Geometry: final body of the model. Coordinates: model frame, mm. A direction names the side the tool comes from. Give positions to 0.01 mm unless a question says otherwise; leave off trailing zeros. Write each loop counter-clockwise with the first axis right and the second up, starting at its lowest first coordinate (ties: lowest second). Pieces come first, ordered by that corner, then holes. Notation, with made-up numbers: M -15.5,32 L -8.5,32 A26 ccw -8.5,59 Z; hole C 80.5,39 d10. An arc over 180 degrees is marked long. Use a Markdown table: item, result. Add a question column.
1) Section B-B on z = 2.75. Return the cut outline in (x, y), then the cut area to 3 significant figures.
2) Pin query (flat end, axial travel): pin 1 (0.6 mm diameter, centred on x = -30, z = 11.5, fed in from +Y) (3 decimals); pin 2 (12 mm diameter, centred on x = -4.5, z = 7, fed in from -Y); pin 3 (0.9 mm diameter, centred on x = -22.5, z = 18.5, fed in from +Y); pin 4 (2.5 mm diameter, centred on y = 6, z = 16.5, fed in from -X). Return the tip coordinate at first contact, or that it passes through.
3) Line query: line 1 (Z direction, x = -24.95, y = 6.5); line 2 (Z direction, x = -2.75, y = 4.5); line 3 (X direction, y = 6.5, z = 13). Output: solid intervals per line, ascending.
4) Section C-C on x = -2.75. Return the cut outline in (y, z), then the cut area to 3 significant figures.
5) Draft query along Z for faces 4 (the flat face through (-8.25, 5, -1)), 5 (the flat face through (-21, 5, 19.05)), 6 (the cylindrical face through (-2.425, 5.053, 14.514)). Return one class per face: +Z half, -Z half, draft (parallel to the pull), parting line (faces both ways), or undercut.
6) Section D-D on y = 1.5. Return the cut outline in (x, z), then the cut area to 3 significant figures.
7) Section A-A on x = -24.95. Return the cut outline in (y, z), then the cut area to 3 significant figures.
8) Set-up query: faces 1 (the flat face through (-31.7, 8.7, 11.4)), 2 (the flat face through (-16, 9.125, 18)), 3 (the flat face through (-35.6, 1.95, 11.4)). Return all of +Z, -Z, +X, -X, +Y, -Y with unobstructed straight access to the full face (end or side cutting, diameter ignored); none if empty.
Autodesk Inventor part; units mm, degrees
ref_plane "YZ Plane" through (0, 0, 0) normal (1, 0, 0) x (0, 1, 0)
ref_plane "XZ Plane" through (0, 0, 0) normal (0, 1, 0) x (-1, 0, 0)
ref_plane "XY Plane" through (0, 0, 0) normal (0, 0, 1) x (1, 0, 0)
sketch "Sketch1" plane through (0, 0, 0) normal (0, 1, 0) x (-1, 0, 0)
  circle A0 centre (2.75, 13.05) radius 1.5
  circle A1 centre (24.95, 2.75) radius 1.5
  line L0 (2, 15.8) -> (25.7, 15.8)
  line L1 (27.7, 13.8) -> (27.7, 2)
  line L2 (25.7, 0) -> (2, 0)
  line L3 (0, 2) -> (0, 13.8)
  arc A2 (0, 2) -> (2, 0) centre (2, 2) ccw
  arc A3 (25.7, 0) -> (27.7, 2) centre (25.7, 2) ccw
  arc A4 (27.7, 13.8) -> (25.7, 15.8) centre (25.7, 13.8) ccw
  arc A5 (2, 15.8) -> (0, 13.8) centre (2, 13.8) ccw
  point P0 (0, 0)
  point P1 (0, 0)
  point P2 (0, 0)
  dimension "d0" = 10.3
  dimension "d1" = 22.2
  dimension "d2" = 2.75
  dimension "d3" = 2.75
  dimension "d4" = 2.75
  dimension "d5" = 2.75
  dimension "d6" = 3
  dimension "d7" = 2
extrude "Extrusion1" add sketch "Sketch1" along normal blind 10.25
sketch "Sketch2" plane through (-2, 0, 0) normal (0, 0, -1) x (-1, 0, 0)
  line L0 (0, 0) -> (23.7, 0)
  line L1 (0, 10.25) -> (23.7, 10.25)
  line L2 (0, 0) -> (0, 10.25)
  line L3 (3.5, 7.25) -> (6.25, 7.25)
  line L4 (6.25, 7.25) -> (6.25, 3)
  line L5 (6.25, 3) -> (3.5, 3)
  line L6 (3.5, 3) -> (3.5, 7.25)
  point P0 (-2, 0)
  dimension "d10" = 4.25
  dimension "d12" = 2.75
  dimension "d13" = 3
  dimension "d14" = 3
  dimension "d15" = 3.5
extrude "Extrusion2" add sketch "Sketch2" along normal blind 2.5
sketch "Sketch3" plane through (-27.7, 0, 2) normal (-1, 0, 0) x (0, 0, 1)
  line L0 (0, 0) -> (11.8, 0)
  line L1 (0, 10.25) -> (11.8, 10.25)
  line L2 (9, 9.125) -> (9.8, 9.125)
  line L3 (9.8, 9.125) -> (9.8, 1.125)
  line L4 (9.8, 1.125) -> (9, 1.125)
  line L5 (9, 1.125) -> (9, 9.125)
  line L6 (-2, 0) -> (-2, 10.25)
  dimension "d18" = 8
  dimension "d20" = 0.8
  dimension "d21" = 1.125
  dimension "d22" = 1.125
  dimension "d23" = 11
extrude "Extrusion3" add sketch "Sketch3" along normal blind 12
sketch "Sketch5" plane through (-25.7, 0, 15.8) normal (0, 0, 1) x (1, 0, 0)
  line L0 (0, 0) -> (23.7, 0)
  line L1 (23.7, 0) -> (23.7, 10.25)
  line L2 (0, 10.25) -> (23.7, 10.25)
  line L3 (9.5, 9.125) -> (10.3, 9.125)
  line L4 (10.3, 9.125) -> (10.3, 1.125)
  line L5 (10.3, 1.125) -> (9.5, 1.125)
  line L6 (9.5, 1.125) -> (9.5, 9.125)
  line L7 (0, 0) -> (0, 10.25)
  point P0 (25.7, 0)
  dimension "d29" = 8
  dimension "d31" = 0.8
  dimension "d33" = 1.125
  dimension "d34" = 1.125
  dimension "d49" = 9.5
  dimension "d50" = 13.4
extrude "Extrusion5" add sketch "Sketch5" along normal blind 3.25 contours L3 L4 L5 L6
sketch "Sketch6" plane through (-15.4, 1.125, 15.8) normal (1, 0, 0) x (0, 0, -1)
  line L0 (0, 0) -> (-3.25, 0)
  line L1 (-3.25, 8) -> (-2.45, 8)
  line L2 (-2.45, 8) -> (-2.45, 0)
  line L3 (-2.45, 0) -> (-3.25, 0)
  line L4 (-3.25, 0) -> (-3.25, 8)
  point P0 (15.8, -1.125)
  dimension "d37" = 0.8
extrude "Extrusion6" add sketch "Sketch6" against normal blind 11
fillet "Fillet1" radius 1 1 edges at (-15.4, 5.125, 19.05)
fillet "Fillet2" radius 0.25 1 edges at (-16.2, 5.125, 18.25)
sketch "Sketch9" plane through (-25.7, 0, 19.05) normal (0, 0, 1) x (1, 0, 0)
  line L0 (9.3, 9.125) -> (-0.7, 9.125)
  line L1 (-0.7, 1.125) -> (-0.7, 9.125)
  line L2 (9.3, 1.125) -> (-0.7, 1.125)
  line L3 (7.3, 9.125) -> (7.3, 8.3)
  line L4 (7.3, 8.3) -> (-0.7, 8.3)
  line L5 (7.3, 1.125) -> (7.3, 1.95)
  line L6 (7.3, 1.95) -> (-0.7, 1.95)
  line L7 (10.3, 1.125) -> (10.3, 9.125)
  point P0 (25.7, 0)
  dimension "d51" = 6.35
  dimension "d53" = 3
extrude "Extrusion9" cut sketch "Sketch9" against normal up to next
sketch "Sketch10" plane through (-27.7, 1.125, 11.8) normal (0, 0, 1) x (1, 0, 0)
  line L0 (0, 8) -> (-12, 8)
  line L1 (-12, 0) -> (-12, 8)
  line L2 (0, 0) -> (-12, 0)
  line L3 (-12, 7.175) -> (-4, 7.175)
  line L4 (-4, 7.175) -> (-4, 8)
  line L5 (-4, 0) -> (-4, 0.825)
  line L6 (-4, 0.825) -> (-12, 0.825)
  point P0 (27.7, -1.125)
  dimension "d56" = 6.35
  dimension "d57" = 8
extrude "Extrusion10" cut sketch "Sketch10" against normal up to next
equation "\"d3\" = d2"
equation "\"d4\" = d2"
equation "\"d5\" = d2"
equation "\"d13\" = d14"
equation "\"d21\" = d22"
equation "\"d33\" = d34"
properties part number "EndStop_LimitSwitch"
Found:
| question | item | result |
|---|---|---|
| 1 | outline | M -27.7,0 L -26.45,0 L -26.45,10.25 L -27.7,10.25 Z; M -23.45,0 L 0,0 L 0,10.25 L -23.45,10.25 Z |
| 1 | area | 253 mm² |
| 2 | pin 1 | y = 9.125 |
| 2 | pin 2 | y = 0 |
| 2 | pin 3 | y = 8.3 |
| 2 | pin 4 | x = -27.08 |
| 3 | line 1 | 0 to 1.25, 4.25 to 15.8, 18.25 to 19.05 |
| 3 | line 2 | 0 to 11.55, 14.55 to 15.8 |
| 3 | line 3 | -27.7 to -4.25, -1.25 to 0 |
| 4 | outline | M 0,0 L 10.25,0 L 10.25,11.55 L 0,11.55 Z; M 0,14.55 L 10.25,14.55 L 10.25,15.8 L 0,15.8 Z |
| 4 | area | 131 mm² |
| 5 | face 4 | draft |
| 5 | face 5 | +Z half |
| 5 | face 6 | undercut |
| 6 | outline | M -31.7,11 L -27.7,11 L -27.7,2 A2 ccw -25.7,0 L -2,0 A2 ccw 0,2 L 0,13.8 A2 ccw -2,15.8 L -15.4,15.8 L -15.4,18.05 A1 ccw -16.4,19.05 L -18.4,19.05 L -18.4,18.25 L -16.45,18.25 A0.25 cw -16.2,18 L -16.2,15.8 L -25.7,15.8 A2 ccw -27.7,13.8 L -27.7,11.8 L -31.7,11.8 Z; hole C -24.95,2.75 d3; hole C -2.75,13.05 d3 |
| 6 | area | 427 mm² |
| 7 | outline | M 0,0 L 10.25,0 L 10.25,1.25 L 0,1.25 Z; M 0,4.25 L 10.25,4.25 L 10.25,15.8 L 0,15.8 Z; M 1.95,18.25 L 8.3,18.25 L 8.3,19.05 L 1.95,19.05 Z |
| 7 | area | 136 mm² |
| 8 | face 1 | +Z, -Z, -X, +Y |
| 8 | face 2 | +Z, +X, -X, +Y |
| 8 | face 3 | +Z, -Z, -X, -Y |
